Work out the finished part from the listing and answer in its coordinate system (mm). Give positions to 0.01 mm unless a question says otherwise; leave off trailing zeros. Write each loop counter-clockwise with the first axis right and the second up, starting at its lowest first coordinate (ties: lowest second). Pieces come first, ordered by that corner, then holes. Notation, with made-up numbers: (-31.75, -6) - (19.25, -6) arc R22 ccw to (19.25, 4) - close; hole circle Ø3 at (45, 86.5). An arc over 180 degrees is marked (long way). Write item = value, one per line.
Autodesk Inventor part; units mm, degrees
ref_plane "YZ Plane" through (0, 0, 0) normal (1, 0, 0) x (0, 1, 0)
ref_plane "XZ Plane" through (0, 0, 0) normal (0, 1, 0) x (-1, 0, 0)
ref_plane "XY Plane" through (0, 0, 0) normal (0, 0, 1) x (1, 0, 0)
sketch "Sketch1" plane through (0, 0, 0) normal (0, 0, 1) x (1, 0, 0)
  line L0 (-88.9, -92.075) -> (-88.9, 92.075)
  line L1 (-88.9, 92.075) -> (88.9, 92.075)
  line L2 (88.9, 92.075) -> (88.9, -92.075)
  line L3 (88.9, -92.075) -> (-88.9, -92.075)
  line L4 (-88.9, -92.075) -> (88.9, 92.075) construction
  line L5 (-88.9, 92.075) -> (88.9, -92.075) construction
  line L6 (-2.54, 53.34) -> (2.54, 53.34) construction
  line L7 (2.54, 78.74) -> (-2.54, 78.74) construction
  line L8 (-12.7, 63.5) -> (-12.7, 68.58) construction
  line L9 (12.7, 68.58) -> (12.7, 63.5) construction
  line L10 (-2.54, 63.5) -> (-12.7, 63.5) construction
  line L11 (-2.54, 63.5) -> (-2.54, 53.34) construction
  line L12 (-2.54, 78.74) -> (-2.54, 68.58) construction
  line L13 (-12.7, 68.58) -> (-2.54, 68.58) construction
  line L14 (2.54, 68.58) -> (12.7, 68.58) construction
  line L15 (12.7, 63.5) -> (2.54, 63.5) construction
  line L16 (2.54, 53.34) -> (2.54, 63.5) construction
  line L17 (2.54, 68.58) -> (2.54, 78.74) construction
  circle A0 centre (25.4, 85.725) radius 1.4605
  line L18 (12.7, 66.04) -> (-12.7, 66.04) construction
  line L19 (0, 53.34) -> (0, 78.74) construction
  circle A1 centre (25.4, 46.355) radius 1.4605
  circle A2 centre (-25.4, 85.725) radius 1.4605
  circle A3 centre (-25.4, 46.355) radius 1.4605
  line L20 (12.7, 50.165) -> (-12.7, 50.165)
  line L21 (-12.7, 50.165) -> (-12.7, 45.085)
  line L22 (-12.7, 45.085) -> (12.7, 45.085)
  line L23 (12.7, 45.085) -> (12.7, 50.165)
  line L24 (12.7, 50.165) -> (-12.7, 45.085) construction
  line L25 (-12.7, 50.165) -> (12.7, 45.085) construction
  line L26 (2.54, 60.325) -> (-2.54, 60.325)
  line L27 (-2.54, 60.325) -> (-2.54, 34.925)
  line L28 (-2.54, 34.925) -> (2.54, 34.925)
  line L29 (2.54, 34.925) -> (2.54, 60.325)
  line L30 (2.54, 60.325) -> (-2.54, 34.925) construction
  line L31 (-2.54, 60.325) -> (2.54, 34.925) construction
  circle A4 centre (22.225, 52.4607) radius 2.4384
  circle A5 centre (0, 74.6857) radius 2.4384
  circle A6 centre (-22.225, 52.4607) radius 2.4384
  line L32 (7.62, -36.5282) -> (12.7, -36.5282)
  line L33 (12.7, -36.5282) -> (12.7, -11.1282)
  line L34 (12.7, -11.1282) -> (12.7, -6.2879)
  line L35 (7.62, -6.2879) -> (12.7, -6.2879)
  line L36 (2.54, -6.2879) -> (7.62, -6.2879)
  line L37 (-2.54, -6.2879) -> (2.54, -6.2879)
  line L38 (-7.62, -6.2879) -> (-2.54, -6.2879)
  line L39 (-7.62, -11.1282) -> (-7.62, -6.2879)
  line L40 (-7.62, -36.5282) -> (-7.62, -11.1282)
  line L41 (-2.54, -36.5282) -> (2.54, -36.5282)
  line L42 (-7.62, -36.5282) -> (-2.54, -36.5282)
  line L43 (2.54, -36.5282) -> (7.62, -36.5282)
  line L44 (15.24, -3.7479) -> (15.24, -11.1282)
  line L45 (15.24, -11.1282) -> (15.24, -39.0682)
  line L46 (15.24, -39.0682) -> (7.62, -39.0682)
  line L47 (7.62, -39.0682) -> (2.54, -39.0682)
  line L48 (2.54, -39.0682) -> (-2.54, -39.0682)
  line L49 (-2.54, -39.0682) -> (-10.16, -39.0682)
  line L50 (-10.16, -39.0682) -> (-10.16, -11.1282)
  line L51 (-10.16, -11.1282) -> (-10.16, -3.7479)
  line L52 (-10.16, -3.7479) -> (-2.54, -3.7479)
  line L53 (-2.54, -3.7479) -> (2.54, -3.7479)
  line L54 (2.54, -3.7479) -> (7.62, -3.7479)
  line L55 (7.62, -3.7479) -> (15.24, -3.7479)
  line L56 (-38.1, -27.758) -> (43.18, -27.758)
  line L57 (43.18, -27.758) -> (43.18, -15.058)
  line L58 (43.18, -15.058) -> (-38.1, -15.058)
  line L59 (-38.1, -15.058) -> (-38.1, -27.758)
  line L60 (-38.1, -27.758) -> (43.18, -15.058) construction
  line L61 (43.18, -27.758) -> (-38.1, -15.058) construction
  line L62 (-38.1, -27.758) -> (-38.1, -92.075)
  line L63 (43.18, -27.758) -> (43.18, -92.075)
  point P0 (0, 0)
  point P1 (0, 47.625)
  point P2 (2.54, 50.165)
  point P3 (2.54, 45.085)
  point P4 (-2.54, 45.085)
  point P5 (-2.54, 50.165)
  point P6 (2.54, -21.408)
  point P7 (2.54, -21.408)
  point P8 (-10.16, -27.758)
  point P9 (-10.16, -15.058)
  point P10 (15.24, -15.058)
  point P11 (15.24, -27.758)
  dimension "d0" = 184.15
  dimension "d1" = 177.8
  dimension "d26" = 5.08
  dimension "d27" = 5.08
  dimension "d28" = 6.35
  dimension "d29" = 2.921
  dimension "d30" = 63.5
  dimension "d31" = 25.4
  dimension "d32" = 25.4
  dimension "d33" = 25.4
  dimension "d34" = 5.08
  dimension "d35" = 5.08
  dimension "d36" = 44.45
  dimension "d37" = 88.9
  dimension "d40" = 2.54
  dimension "d41" = 81.28
  dimension "d42" = 12.7
  dimension "d43" = 30.2403
  dimension "d44" = 15.1201
extrude "Extrusion1" add sketch "Sketch1" along normal mid plane 5.08 contours L0 L1 L2 L3 L63 L57 L58 L45 L44 L55 L54 L53 L52 L51 L50 L59 L62
sketch "Sketch2" plane through (0, 0, 2.54) normal (0, 0, 1) x (1, 0, 0)
  circle A0 centre (-22.86, -3.175) radius 1.4605 construction
  circle A1 centre (-12.7, -3.175) radius 1.4605 construction
  line L0 (0, -6.35) -> (0, 0) construction
  line L1 (-25.4, 0) -> (0, 0) construction
  line L2 (-25.4, 0) -> (-25.4, -6.35) construction
  line L3 (0, -6.35) -> (-25.4, -6.35) construction
  line L4 (15.24, -6.35) -> (15.24, 0) construction
  line L5 (0, 0) -> (15.24, 0) construction
  line L6 (0, -6.35) -> (0, 0) construction
  line L7 (15.24, -6.35) -> (0, -6.35) construction
  line L8 (69.088, -61.595) -> (69.088, -46.355)
  line L9 (69.088, -46.355) -> (75.438, -46.355)
  line L10 (75.438, -46.355) -> (75.438, -61.595)
  line L11 (75.438, -86.995) -> (69.088, -86.995) construction
  line L12 (88.9, -92.075) -> (88.9, 92.075)
  line L13 (-88.9, -92.075) -> (88.9, -92.075)
  line L14 (69.088, -61.595) -> (75.438, -61.595)
  circle A2 centre (72.263, -84.455) radius 1.4605
  circle A3 centre (72.263, -69.215) radius 1.4605
  point P0 (-25.4, -3.175)
  dimension "d14" = 13.462
  dimension "d15" = 6.35
  dimension "d16" = 5.08
  dimension "d17" = 40.64
  dimension "d18" = 15.24
  dimension "d19" = 2.921
  dimension "d20" = 2.921
  dimension "d21" = 15.24
  dimension "d22" = 3.175
  dimension "d23" = 2.54
extrude "Extrusion2" cut sketch "Sketch2" against normal through all
mirror "Mirror1" about plane through (0, 0, 0) normal (1, 0, 0) of "Extrusion2"
sketch "Sketch7" plane through (0, 0, 2.54) normal (0, 0, 1) x (1, 0, 0)
  circle A0 centre (-72.263, -84.455) radius 1.4605
  line L0 (-69.088, -61.595) -> (-75.438, -61.595)
  line L1 (-75.438, -61.595) -> (-75.438, -46.355)
  line L2 (-75.438, -46.355) -> (-69.088, -46.355)
  line L3 (-69.088, -46.355) -> (-69.088, -61.595)
  circle A1 centre (-72.263, -69.215) radius 1.4605
  circle A2 centre (72.263, -84.455) radius 1.4605
  circle A3 centre (72.263, -69.215) radius 1.4605
  line L4 (69.088, -46.355) -> (75.438, -46.355)
  line L5 (75.438, -46.355) -> (75.438, -61.595)
  line L6 (75.438, -61.595) -> (69.088, -61.595)
  line L7 (69.088, -61.595) -> (69.088, -46.355)
  line L8 (15.24, -3.7479) -> (15.24, -15.058)
  line L9 (15.24, -15.058) -> (43.18, -15.058)
  line L10 (43.18, -15.058) -> (43.18, -92.075)
  line L11 (-10.16, -15.058) -> (-10.16, -3.7479)
  line L12 (-38.1, -92.075) -> (-38.1, -15.058)
  line L13 (-38.1, -15.058) -> (-10.16, -15.058)
  line L14 (-10.16, -3.7479) -> (15.24, -3.7479)
  circle A4 centre (-22.225, 52.4607) radius 2.4384
  circle A5 centre (0, 74.6857) radius 2.4384
  circle A6 centre (22.225, 52.4607) radius 2.4384
  circle A7 centre (25.4, 85.725) radius 1.4605
  circle A8 centre (25.4, 46.355) radius 1.4605
  circle A9 centre (-25.4, 85.725) radius 1.4605
  circle A10 centre (-25.4, 46.355) radius 1.4605
  line L15 (-12.7, 45.085) -> (-12.7, 50.165)
  line L16 (-12.7, 50.165) -> (-2.54, 50.165)
  line L17 (-2.54, 50.165) -> (-2.54, 60.325)
  line L18 (-2.54, 60.325) -> (2.54, 60.325)
  line L19 (2.54, 60.325) -> (2.54, 50.165)
  line L20 (2.54, 50.165) -> (12.7, 50.165)
  line L21 (12.7, 50.165) -> (12.7, 45.085)
  line L22 (12.7, 45.085) -> (2.54, 45.085)
  line L23 (2.54, 45.085) -> (2.54, 34.925)
  line L24 (2.54, 34.925) -> (-2.54, 34.925)
  line L25 (-2.54, 34.925) -> (-2.54, 45.085)
  line L26 (-2.54, 45.085) -> (-12.7, 45.085)
  line L27 (-88.9, -92.075) -> (-38.1, -92.075)
  line L28 (88.9, -92.075) -> (88.9, 92.075)
  line L29 (88.9, 92.075) -> (-88.9, 92.075)
  line L30 (-88.9, 92.075) -> (-88.9, -92.075)
  line L31 (43.18, -92.075) -> (88.9, -92.075)
  point P0 (0, 0)
sketch "Sketch8" plane through (0, 0, 2.54) normal (0, 0, 1) x (1, 0, 0)
  line L0 (-57.15, -92.075) -> (-38.1, -53.975)
  line L1 (0, 0) -> (0, -92.075) construction
  line L2 (-88.9, -92.075) -> (-38.1, -92.075)
  line L3 (-38.1, -92.075) -> (-38.1, -15.058)
  line L4 (-57.15, -92.075) -> (-38.1, -92.075)
  line L5 (43.18, -15.058) -> (43.18, -92.075)
  line L6 (43.18, -92.075) -> (62.23, -92.075)
  line L7 (43.18, -92.075) -> (88.9, -92.075)
  line L8 (62.23, -92.075) -> (43.18, -53.975)
  line L9 (43.18, -53.975) -> (43.18, -92.075)
  dimension "d45" = 19.05
  dimension "d46" = 38.1
  dimension "d47" = 19.05
  dimension "d48" = 38.1
extrude "Extrusion3" cut sketch "Sketch8" against normal blind 25.4
sketch "Sketch9" plane through (0, 0, 2.54) normal (0, 0, 1) x (1, 0, 0)
  line L0 (-88.9, 92.075) -> (88.9, 92.075)
  line L1 (50.8, 92.075) -> (88.9, 53.975)
  line L2 (88.9, 53.975) -> (88.9, 92.075)
  line L3 (88.9, 92.075) -> (50.8, 92.075)
  line L4 (-88.9, -92.075) -> (-88.9, 92.075)
  line L5 (-88.9, 92.075) -> (-88.9, 53.975)
  line L6 (-50.8, 92.075) -> (-88.9, 53.975)
  line L7 (-88.9, 92.075) -> (-50.8, 92.075)
  point P0 (0, 0)
  dimension "d51" = 38.1
  dimension "d52" = 38.1
  dimension "d53" = 38.1
extrude "Extrusion4" cut sketch "Sketch9" against normal blind 25.4
properties part number "BoardProj"
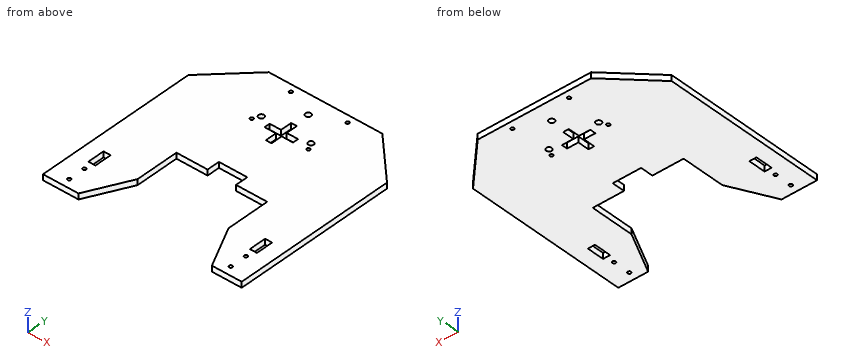
1. Find section C-C, the plane y = -75.5. Give the vertices of the cut face in (x, z), then the cut area to 3 significant figures.
Solution:
outline = (-88.9, -2.54) - (-48.86, -2.54) - (-48.86, 2.54) - (-88.9, 2.54) - close; (53.94, -2.54) - (88.9, -2.54) - (88.9, 2.54) - (53.94, 2.54) - close
area = 381 mm^2
2. Find section B-B, the plane x = 0. Give the vertices of the cut face in (y, z) (3 decimals), then the cut area to 3 significant figures.
Solution:
outline = (-3.748, -2.54) - (34.925, -2.54) - (34.925, 2.54) - (-3.748, 2.54) - close; (60.325, -2.54) - (72.247, -2.54) - (72.247, 2.54) - (60.325, 2.54) - close; (77.124, -2.54) - (92.075, -2.54) - (92.075, 2.54) - (77.124, 2.54) - close
area = 333 mm^2
3. Straight lines are drawn through the part: line 1 (Y direction, x = 25.4, z = -1) (1 decimal); line 2 (Y direction, x = 10, z = -0.4) (3 decimals); line 3 (Y direction, x = 34.5, z = -1.9) (3 decimals). For each, find the intervals that lie inside material, in ascending order.
Solution:
line_1 = -15.1 to 44.9, 47.8 to 84.3, 87.2 to 92.1
line_2 = -3.748 to 45.085, 50.165 to 92.075
line_3 = -15.058 to 92.075
4. Find section A-A, the plane y = -23. Give the vertices of the cut face in (x, z).
Solution:
outline = (-88.9, -2.54) - (-38.1, -2.54) - (-38.1, 2.54) - (-88.9, 2.54) - close; (43.18, -2.54) - (88.9, -2.54) - (88.9, 2.54) - (43.18, 2.54) - close
5. Given pin 1 (8 mm diameter, centred on x = -22.22, y = 52.46, fed in from +Z), flat-ended and moving along its own axis, determine where the tip first touches the part or whether it passes through.
Solution:
pin_1 = 2.54
6. Find section D-D, the plane z = 0.8. Give the number of separate pieces and of enclosed holes in the cut face, then the cut area to 3 significant figures.
Solution:
separate_pieces = 1
enclosed_holes = 14
area = 23,500 mm^2
